Design review of the part built by this model. Coordinates are the model's own, in mm. A direction names the side the tool comes from. Round coordinates to 2 decimals unless told otherwise and drop trailing zeros. Write each loop counter-clockwise with the first axis right and the second up, starting at its lowest first coordinate (ties: lowest second). Pieces come first, ordered by that corner, then holes. Notation, with made-up numbers: (-34, 81) -> (-3, 81) arc R19 cw to (-3, 113) -> close; hole circle Ø8 at (88, 83). An arc over 180 degrees is marked (long way). Write item = value, one per line. Start each with the question number.
Item 1: Add section B-B, the plane x = 5. State the section outline as (y, z) points.
Item 2: Mouldability with a two-part tool opening along Y and no side actions: class faces 1 (the cylindrical face through (3.243, 33.226, -13.39)), 2 (the cylindrical face through (65.01, 34.14, -56.1)), 3 (the flat face through (67, 27, -45)) as released by +Y, released by -Y, zero draft, split by the parting line, or undercut.
Item 3: To check wall thickness, follow L1, parallel to Y at x = 68, z = -38; L2, parallel to Y at x = 74.5, z = -51.5; L3, parallel to X at y = 23.5, z = -4. State the ranges of each line that lie inside material, in increasing order.
Item 4: Add section D-D, the plane y = 12. State the section outline as (x, z) points, then the cut area to 3 significant figures.
Item 5: Machinability: for faces 4 (the flat face through (65, 23, -30)), 5 (the flat face through (45, 30.2, -17.929)), 6 (the flat face through (4, 32, -17.929)), 7 (the flat face through (39.071, 33, -26)), 8 (the flat face through (6, 31.5, -11)), which of the approach directions +Z, -Z, +X, -X, +Y, -Y give a long, thin tool a straight path to every point of the face, cutting with its end or side? Answer none if there is none.
Item 6: Add section A-A, the plane x = 76.5. State the section outline as (y, z) points, then the cut area to 3 significant figures.
Item 7: Add section C-C, the plane z = -30.5. State the section outline as (x, y) points, then the cut area to 3 significant figures.
Item 8: For pin 1 Ø4 at (x, y) = (4.5, 32) entering from -Z; pin 2 Ø2 at (x, y) = (71.25, 15.54) entering from +Z; pin 3 Ø2.5 at (y, z) = (33.5, -27.5) entering from -X; pin 4 Ø6 at (x, z) = (36, -44) entering from -Y, all flat-tipped, find the tip position at first contact; note any pin that passes through.
from build123d import *

# Parameters (mm, degrees)
SKETCH1_R               = 1.8
BOSS_EXTRUDE1_DEPTH     = 35
CUT_EXTRUDE1_DEPTH      = 20
FILLET1_R               = 3
CUT_EXTRUDE2_DEPTH      = 102.662431606
CUT_EXTRUDE2_DEPTH_BACK = 102.662431606
SKETCH5_W               = 48
SKETCH5_H               = 48
CUT_EXTRUDE3_DEPTH      = 30
SKETCH6_W               = 30.142
SKETCH6_H               = 9
CUT_EXTRUDE4_DEPTH      = 31.4
SKETCH7_W               = 21
SKETCH7_H               = 9
CUT_EXTRUDE5_DEPTH      = 85.173689476
SKETCH8_R               = 3.5
CUT_EXTRUDE6_DEPTH      = 1.5
SKETCH11_R              = 1.75
SKETCH11_R_2            = 5.5
BOSS_EXTRUDE3_DEPTH     = 10


with BuildPart() as part:
    # Sketch1 → Boss-Extrude1 (new body)
    with BuildSketch(Plane(origin=(0, 0, 0), x_dir=(1, 0, 0), z_dir=(0, 1, 0))):
        Polygon((6.964635103, 17.928932188), (0, 17.928932188), (0, 0), (82.5, 0), (82.5, 57), (48, 57), (48, 48), (32, 48), (32, 41), (39.071067812, 33.928932188), (39.071067812, 17.928932188), (35.071067812, 17.928932188), (28.517851458, 13.340320697), (13.517851458, 13.340320697), align=None)
        with Locations(Location((36, 44, 0), (0, 0, 270))):
            Circle(SKETCH1_R, mode=Mode.SUBTRACT)
        with Locations(Location((36, 13, 0), (0, 0, 270))):
            Circle(SKETCH1_R, mode=Mode.SUBTRACT)
        with Locations(Location((5, 13, 0), (0, 0, 270))):
            Circle(SKETCH1_R, mode=Mode.SUBTRACT)
    extrude(amount=BOSS_EXTRUDE1_DEPTH)

    # Sketch2 → Cut-Extrude1 (cut)
    with BuildSketch(Plane.XZ):
        Polygon((82.5, -57), (82.5, 0), (67, 0), (67, -48), (48, -48), (48, -57), align=None)
    extrude(amount=-CUT_EXTRUDE1_DEPTH, mode=Mode.SUBTRACT)

    # Fillet1
    fillet1_edges = [part.edges().sort_by_distance(p)[0] for p in [
        (65.25, 35, -57),
        (65.25, 20, -57),
    ]]
    fillet(fillet1_edges, radius=FILLET1_R)

    # Sketch3 → Cut-Extrude2 (cut, two sides: drawn at the far end of the back side and taken through both)
    with BuildSketch(Plane(origin=(0, 0, -48), x_dir=(-1, 0, 0), z_dir=(0, 0, -1)).offset(-CUT_EXTRUDE2_DEPTH_BACK)):
        with BuildLine():
            ThreePointArc((-50.010278489, 9.892519672), (-64.998857714, 9.630893048), (-50.028539764, 8.846331929))
            Line((-50.028539764, 8.846331929), (-48.036150368, 8.672020444))
            ThreePointArc((-48.036150368, 8.672020444), (-51.081893028, 2.4958653), (-57.5, 0))
            Line((-57.5, 0), (-48, 0))
            Line((-48, 0), (-48, 9.997873903))
            Line((-48, 9.997873903), (-50.010278489, 9.892519672))
        make_face()
        with BuildLine():
            Line((-67, 0), (-57.5, 0))
            ThreePointArc((-57.5, 0), (-64.217514421, 2.782485579), (-67, 9.5))
            Line((-67, 9.5), (-67, 0))
        make_face()
    extrude(amount=CUT_EXTRUDE2_DEPTH + CUT_EXTRUDE2_DEPTH_BACK, mode=Mode.SUBTRACT)

    # Sketch5 → Cut-Extrude3 (cut)
    with BuildSketch(Plane.XZ):
        with Locations((24, -24)):
            Rectangle(SKETCH5_W, SKETCH5_H)
    extrude(amount=-CUT_EXTRUDE3_DEPTH, mode=Mode.SUBTRACT)

    # Sketch6 → Cut-Extrude4 (cut)
    with BuildSketch(Plane(origin=(82.5, 0, 0), x_dir=(0, 0, -1), z_dir=(1, 0, 0))):
        with Locations((29.929, 27.5)):
            Rectangle(SKETCH6_W, SKETCH6_H)
    extrude(amount=-CUT_EXTRUDE4_DEPTH, mode=Mode.SUBTRACT)

    # Sketch7 → Cut-Extrude5 (cut, through all)
    with BuildSketch(Plane(origin=(51.1, 0, 0), x_dir=(0, 0, -1), z_dir=(1, 0, 0))):
        with Locations((28.428932188, 27.5)):
            Rectangle(SKETCH7_W, SKETCH7_H)
    extrude(amount=-CUT_EXTRUDE5_DEPTH, mode=Mode.SUBTRACT)

    # Sketch8 → Cut-Extrude6 (cut)
    with BuildSketch(Plane.XZ.offset(-30)):
        with Locations(Location((5, -13, 0), (0, 0, 270))):
            Circle(SKETCH8_R)
        with Locations(Location((36, -13, 0), (0, 0, 270))):
            Circle(SKETCH8_R)
        with Locations(Location((36, -44, 0), (0, 0, 270))):
            Circle(SKETCH8_R)
    extrude(amount=-CUT_EXTRUDE6_DEPTH, mode=Mode.SUBTRACT)

    # Sketch11 → Boss-Extrude3 (add)
    with BuildSketch(Plane.XY):
        with BuildLine():
            Line((67, 20), (67, 9.5))
            ThreePointArc((67, 9.5), (66.795496221, 7.539451607), (66.190789474, 5.663311542))
            ThreePointArc((66.190789474, 5.663311542), (83.374491132, 0.912720357), (82.5, 18.719544457))
            Line((82.5, 18.719544457), (82.5, 20))
            Line((82.5, 20), (67, 20))
        make_face()
        with Locations((82.537676642, 14.748472232)):
            Circle(SKETCH11_R, mode=Mode.SUBTRACT)
        with Locations((70.462323358, 4.251527768)):
            Circle(SKETCH11_R, mode=Mode.SUBTRACT)
        with Locations((81.748472232, 3.462323358)):
            Circle(SKETCH11_R, mode=Mode.SUBTRACT)
        with Locations((76.5, 9.5)):
            Circle(SKETCH11_R_2, mode=Mode.SUBTRACT)
        with Locations((71.251527768, 15.537676642)):
            Circle(SKETCH11_R, mode=Mode.SUBTRACT)
    extrude(amount=-BOSS_EXTRUDE3_DEPTH)


solid = part.part
Result set:
q1.outline = (30, -17.93) -> (35, -17.93) -> (35, -14.8) -> (31.5, -14.8) -> (31.5, -16.5) -> (30, -16.5) -> close; (30, -9.5) -> (31.5, -9.5) -> (31.5, -11.2) -> (35, -11.2) -> (35, 0) -> (30, 0) -> close
q2.face_1 = zero draft
q2.face_2 = released by +Y
q2.face_3 = undercut
q3.L1 = 20 to 23, 32 to 35
q3.L2 = 20 to 35
q3.L3 = 48 to 82.5
q4.outline = (48, -48) -> (50.43, -48) -> (50.43, 0) -> (48, 0) -> close; (64.57, -48) -> (67, -48) -> (67, -10) -> (71.6, -10) -> (71.6, 0) -> (64.57, 0) -> close; (81.4, -10) -> (87.21, -10) -> (87.21, 0) -> (81.4, 0) -> close
q4.area = 337 mm²
q5.face_4 = +X
q5.face_5 = -X
q5.face_6 = -Z, -X, +Y, -Y
q5.face_7 = -X, +Y, -Y
q5.face_8 = -Y
q6.outline = (-1.5, -10) -> (4, -10) -> (4, 0) -> (-1.5, 0) -> close; (15, -10) -> (20, -10) -> (20, -54) arc R3 ccw to (23, -57) -> (32, -57) arc R3 ccw to (35, -54) -> (35, 0) -> (15, 0) -> close; hole (23, -45) -> (32, -45) -> (32, -14.86) -> (23, -14.86) -> close
q6.area = 685 mm²
q7.outline = (39.07, 32) -> (82.5, 32) -> (82.5, 35) -> (39.07, 35) -> close; (48, 10) -> (50.01, 9.89) arc R7.5 cw (long way) to (50.03, 8.85) -> (48.04, 8.67) arc R9.5 ccw to (67, 9.5) -> (67, 20) -> (82.5, 20) -> (82.5, 23) -> (48, 23) -> close
q7.area = 396 mm²
q8.pin_1 = -17.93
q8.pin_2 = through
q8.pin_3 = 39.07
q8.pin_4 = 31.5
